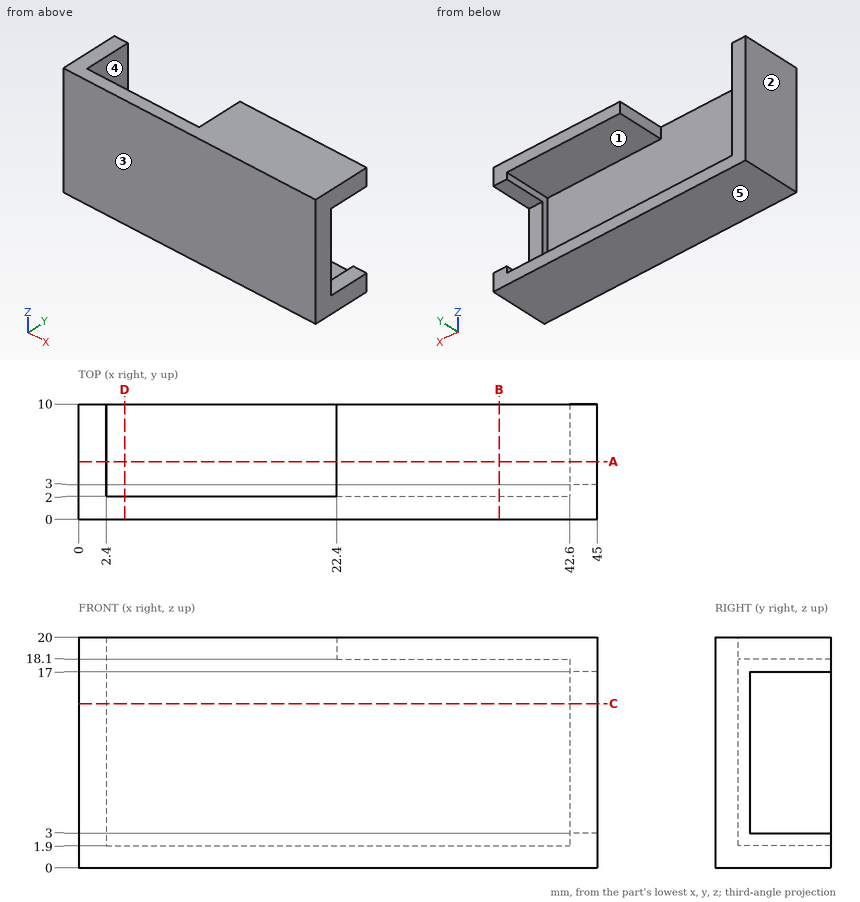
Could you check a few things on this drawing? It's one solid part, dimensions in mm from its lowest x, y, z. A direction names the side the tool comes from. Round coordinates to 2 decimals unless told otherwise and drop trailing zeros. Write each loop counter-clockwise with the first axis right and the second up, starting at its lowest first coordinate (ties: lowest second). Pieces come first, ordered by that corner, then holes. Notation, with made-up numbers: (81, 11.5) -> (109, 11.5) arc R20 cw to (109, 34.5) -> close; hole circle Ø1 at (53.25, 35). An arc over 180 degrees is marked (long way). One line per question, with ' | ' between items. Start each with the question number.
1) On a 3-axis mill with a long thin cutter (end or side, diameter ignored), from which of +Z, -Z, +X, -X, +Y, -Y can I reach the whole of each face in a straight line? I mean the marked faces 4 and 5. Say none if no direction works.
2) I'm going to push flat-ended pins straight in: P1, Ø10, axis at x = 11, z = 14, coming from the +Y side; P2, Ø1.5, axis at x = 14.5, y = 6.5, coming from the +Z side; P3, Ø1.2, axis at x = 44, z = 12.5, coming from the +Y side. Where does each tip first touch, or does it pass through?
3) Suppose I cut it at B-B on x = 36.5. Write out the boundary of the cut face in (y, z), then the cut area to 3 significant figures.
4) If we mould it in two halves opening along X, with no side actions, what happens to the marked faces 1, 2 and 3? For each: released by +X, released by -X, zero draft, split by the parting line, or undercut.
5) Suppose I cut it at D-D on x = 4. Write out the boundary of the cut face in (y, z), then the cut area to 3 significant figures.
6) I need wall thicknesses on line 1 (Z direction, x = 32, y = 4); line 2 (Z direction, x = 20, y = 7.75); line 3 (X direction, y = 7, z = 5.5). Which ranges of each line are inside material? Lowest first, please. Write a range as [from, to].
7) Suppose I cut it at A-A on y = 5. Write out the boundary of the cut face in (x, z), then the cut area to 3 significant figures.
8) Suppose I cut it at C-C on z = 14.25. Write out the boundary of the cut face in (x, y).
Return value:
1) face 4: +Z, +Y | face 5: -Z, +X, -X, +Y, -Y
2) P1: stops at y = 2 | P2: stops at z = 1.9 | P3: stops at y = 3
3) outline: (0, 0) -> (10, 0) -> (10, 1.9) -> (2, 1.9) -> (2, 18.1) -> (10, 18.1) -> (10, 20) -> (0, 20) -> close | area: 70.4 mm2
4) face 1: undercut | face 2: released by -X | face 3: zero draft
5) outline: (0, 0) -> (10, 0) -> (10, 1.9) -> (2, 1.9) -> (2, 20) -> (0, 20) -> close | area: 55.2 mm2
6) line 1: z = [0, 1.9], [18.1, 20] | line 2: z = [0, 1.9] | line 3: x = [0, 2.4]
7) outline: (0, 0) -> (45, 0) -> (45, 3) -> (42.6, 3) -> (42.6, 1.9) -> (2.4, 1.9) -> (2.4, 20) -> (0, 20) -> close; (22.4, 18.1) -> (42.6, 18.1) -> (42.6, 17) -> (45, 17) -> (45, 20) -> (22.4, 20) -> close | area: 177 mm2
8) outline: (0, 0) -> (45, 0) -> (45, 3) -> (42.6, 3) -> (42.6, 2) -> (2.4, 2) -> (2.4, 10) -> (0, 10) -> close
